Verification items for the finished model (mm, model axes). A direction names the side the tool comes from. Round coordinates to 2 decimals unless told otherwise and drop trailing zeros. Order: outer loops, then holes, each group sorted by start corner. A loop starts at its lowest first (then second) coordinate and runs counter-clockwise, first axis right, second up. Notation, with made-up numbers: (57, 0) -> (68, 0) arc R31 cw to (68, 26) -> close; hole circle Ø1 at (9, 55.5). An arc over 180 degrees is marked (long way). Put each result on its own line as item: value.
```python
from build123d import *

# Parameters (mm, degrees)
F1_DEPTH = 12.7


with BuildPart() as f1:
    # F0 (on Front) → F1 (new body)
    with BuildSketch(Plane.XZ):
        with BuildLine():
            Line((-2.8614659345, 25.2383044737), (-152.2392334973, 12.6989824054))
            ThreePointArc((-152.2392334973, 12.6989824054), (-165.0996721713, 0.0912509774), (-152.421732718, -12.6999814051))
            Line((-152.421732718, -12.6999814051), (-2.1237788852, -25.3110561464))
            ThreePointArc((-2.1237788852, -25.3110561464), (25.3973091766, -0.3697114954), (-1.3861233029, 25.3621501886))
            Line((-1.3861233029, 25.3621501886), (-2.8614659345, 25.2383044737))
        make_face()
        with BuildLine():
            ThreePointArc((-1.8591100152, 22.1471066948), (22.2249999045, 0.0020599789), (-1.8550044649, -22.1474509467))
            Line((-1.8550044649, -22.1474509467), (-1.8591100471, -22.1471070753))
            Line((-1.8591100471, -22.1471070753), (-14.1088199902, -21.1211078896))
            Line((-14.1088199902, -21.1211078896), (-144.7998013534, -10.1748209091))
            Line((-144.7998013534, -10.1748209091), (-152.5780849398, -9.5233350647))
            ThreePointArc((-152.5780849398, -9.5233350647), (-161.9234930515, 0.1694257913), (-152.2392334973, 9.5236431649))
            Line((-152.2392334973, 9.5236431649), (-1.8591100152, 22.1471066948))
        make_face(mode=Mode.SUBTRACT)
        with BuildLine():
            ThreePointArc((-1.3861233029, 25.3621501886), (-2.1246971603, 25.3109790798), (-2.8614659345, 25.2383044737))
            Line((-2.8614659345, 25.2383044737), (-1.3861233029, 25.3621501886))
        make_face()
    extrude(amount=F1_DEPTH)


solid = f1.part
```
Item 1: Sectioned sample at C-C, the plane x = -71.5. Record the boundary of the cut face in (y, z), then the cut area to 3 significant figures.
Geometry check:
outline: (-12.7, -19.49) -> (0, -19.49) -> (0, -16.31) -> (-12.7, -16.31) -> close; (-12.7, 16.3) -> (0, 16.3) -> (0, 19.48) -> (-12.7, 19.48) -> close
area: 80.7 mm2
Item 2: Tool access check on faces 1 (the face through (-70, -12.7, -17)), 2 (the face through (-161.925, -6.261, -0.04)). Record the directions out of +Z, -Z, +X, -X, +Y, -Y that give a thin tool (end or side, any length) a straight path to the whole face; none if there is none.
Geometry check:
face 1: +Z, -Z, +X, -X, -Y
face 2: +Y, -Y
Item 3: Material ranges on line 1 along Z through (x, y) = (0, -2.75) (3 decimals); line 2 along X through (y, z) = (-4.75, 0) (3 decimals); line 3 along Z through (x, y) = (-150.5, -0.75), recorded low to high.
Geometry check:
line 1: -25.4 to -22.225, 22.225 to 25.4
line 2: -165.1 to -161.925, 22.225 to 25.4
line 3: -12.86 to -9.7, 9.67 to 12.84
Item 4: Sectioned sample at A-A, the plane z = 0. Record the boundary of the cut face in (x, y) (3 decimals).
Geometry check:
outline: (-165.1, -12.7) -> (-161.925, -12.7) -> (-161.925, 0) -> (-165.1, 0) -> close; (22.225, -12.7) -> (25.4, -12.7) -> (25.4, 0) -> (22.225, 0) -> close
Item 5: Release check for a two-part mould opening along X. For faces 3 (the face through (-78.102, -6.261, 15.747)), 4 (the face through (-70, 0, -17)), 5 (the face through (-78.325, -6.261, -18.917)) record: pulls with the +X half, pulls with the -X half, needs draft (parallel to the pull), parting line crosses it, or undercut.
Geometry check:
face 3: undercut
face 4: needs draft
face 5: pulls with the -X half
Item 6: Depth check by flat-ended pin: pin 1 Ø4 at (x, y) = (-2.5, -5) entering from +Z; pin 2 Ø4 at (x, y) = (-126, -9.5) entering from -Z; pin 3 Ø1.5 at (x, y) = (-54, -8) entering from +Z. Enter the tip coordinate at first touch or a pass-through.
Geometry check:
pin 1: z = 25.4
pin 2: z = -15.08
pin 3: z = 21.01
Item 7: Sectioned sample at B-B, the plane y = -5.5. Record the boundary of the cut face in (x, z) (3 decimals), then the cut area to 3 significant figures.
Geometry check:
outline: (-152.422, -12.7) -> (-2.124, -25.311) arc R25.4 ccw (long way) to (-2.861, 25.238) -> (-152.239, 12.699) arc R12.7 ccw (long way) to start; hole (-152.578, -9.523) -> (-1.855, -22.147) arc R22.225 ccw (long way) to (-1.859, 22.147) -> (-152.239, 9.524) arc R9.525 ccw to start
area: 1,320 mm2
